Build history of the part. All positions in model axes, mm. A direction names the side the tool comes from. Give positions to 0.01 mm unless a question says otherwise; leave off trailing zeros. Write each loop counter-clockwise with the first axis right and the second up, starting at its lowest first coordinate (ties: lowest second). Pieces come first, ordered by that corner, then holes. Notation, with made-up numbers: (51, 28.5) -> (63, 28.5) arc R7 ccw to (63, 39.5) -> close; hole circle Ø4 at (18, -30). An arc over 180 degrees is marked (long way). Put each result on its own line as item: value.
from build123d import *

# Parameters (mm, degrees)
SKETCH1_W           = 100
SKETCH1_H           = 50
BOSS_EXTRUDE1_DEPTH = 50
CUT_EXTRUDE1_REACH  = 88.603
SKETCH2_W           = 40
SKETCH2_H           = 40
CUT_EXTRUDE2_REACH  = 77
SKETCH3_W           = 40
SKETCH3_H           = 40


with BuildPart() as part:
    # Sketch1 → Boss-Extrude1 (new body)
    with BuildSketch(Plane.XY):
        Rectangle(SKETCH1_W, SKETCH1_H)
    extrude(amount=BOSS_EXTRUDE1_DEPTH)

    # Sketch2 → Cut-Extrude1 (cut, up to next)
    with BuildSketch(Plane.XZ.offset(25), mode=Mode.PRIVATE) as cut_extrude1_sk1:
        with Locations((25, 25)):
            Rectangle(SKETCH2_W, SKETCH2_H)
    cut_extrude1_tool1 = extrude(cut_extrude1_sk1.sketch, amount=-CUT_EXTRUDE1_REACH, mode=Mode.PRIVATE) & part.part
    add(cut_extrude1_tool1.solids().sort_by_distance((25, -25, 25))[0], mode=Mode.SUBTRACT)

    # Sketch3 → Cut-Extrude2 (cut, up to next)
    with BuildSketch(Plane.XY.offset(50), mode=Mode.PRIVATE) as cut_extrude2_sk1:
        with Locations((-25, 0)):
            Rectangle(SKETCH3_W, SKETCH3_H)
    cut_extrude2_tool1 = extrude(cut_extrude2_sk1.sketch, amount=-CUT_EXTRUDE2_REACH, mode=Mode.PRIVATE) & part.part
    add(cut_extrude2_tool1.solids().sort_by_distance((-25, 0, 50))[0], mode=Mode.SUBTRACT)


solid = part.part
1) Slice it at A-A (y = -11.5). Write the cut outline in (x, z), plus the area to 3 significant figures.
Filled sheet:
outline: (-50, 0) -> (-45, 0) -> (-45, 50) -> (-50, 50) -> close; (-5, 0) -> (50, 0) -> (50, 50) -> (-5, 50) -> close; hole (5, 5) -> (45, 5) -> (45, 45) -> (5, 45) -> close
area: 1,400 mm2
2) Wall check: L1, parallel to X at y = 2.5, z = 24.5; L2, parallel to Z at x = 20, y = 5; L3, parallel to Y at x = -15, z = 35.5. Give the ranges that are in metal, low to high.
Filled sheet:
L1: -50 to -45, -5 to 5, 45 to 50
L2: 0 to 5, 45 to 50
L3: -25 to -20, 20 to 25
3) Slice it at C-C (x = 21). Write the cut outline in (y, z), plus the area to 3 significant figures.
Filled sheet:
outline: (-25, 0) -> (25, 0) -> (25, 5) -> (-25, 5) -> close; (-25, 45) -> (25, 45) -> (25, 50) -> (-25, 50) -> close
area: 500 mm2
4) Pull direction Y, two halves, no side cores. Call faces 1 (the flat face through (25, 0, 45)), 2 (the flat face through (-12, 25, 25)), 3 (the flat face through (-45, 0, 25)): released by +Y, released by -Y, zero draft, split by the parting line, or undercut.
Filled sheet:
face 1: zero draft
face 2: released by +Y
face 3: undercut
5) Slice it at B-B (z = 32). Write the cut outline in (x, y), plus the area to 3 significant figures.
Filled sheet:
outline: (-50, -25) -> (5, -25) -> (5, 25) -> (-50, 25) -> close; (45, -25) -> (50, -25) -> (50, 25) -> (45, 25) -> close; hole (-45, -20) -> (-5, -20) -> (-5, 20) -> (-45, 20) -> close
area: 1,400 mm2
6) Pin check, flat tip, straight feed: pin 1 (3 mm diameter, centred on x = 19.5, z = 44.5, fed in from +Y). Stop position of the tip, or through.
Filled sheet:
pin 1: y = 25
7) Tool access for faces 4 (the flat face through (-5, 0, 25)), 5 (the flat face through (-50, 0, 25)), 6 (the flat face through (5, 0, 25)): list every direction of +Z, -Z, +X, -X, +Y, -Y with a clear straight run to the whole face (end or side of a thin tool).
Filled sheet:
face 4: +Z, -Z
face 5: +Z, -Z, -X, +Y, -Y
face 6: +Y, -Y
